Source: CAD feature listing. Evaluate the final solid. Frame: model axes, mm. A direction names the side the tool comes from. Give positions to 0.01 mm unless a question says otherwise; leave off trailing zeros. Write each loop counter-clockwise with the first axis right and the second up, starting at its lowest first coordinate (ties: lowest second). Pieces come first, ordered by that corner, then holes. Notation, with made-up numbers: (13.25, -25) - (60.25, -25) arc R25 ccw to (60.25, -3) - close; hole circle Ø7 at (46.25, -13). An arc over 180 degrees is marked (long way). One line per question, with ' | ' between items. Start each with the question number.
(1) Section A-A, the plane y = 6.25. Return loops of the section in (x, z), plus the area to 3 significant figures.
(2) Ray query, line 1 (Y direction, x = -7.75, z = 4); line 2 (Z direction, x = 0, y = 16.25); line 3 (Y direction, x = 1.75, z = 1.25). Return the intervals inside material, ascending. Write a range as [from, to].
(3) Access query for faces 1 (the cylindrical face through (-6, 16, 0)), 2 (the flat face through (0, 5.8, 7)), 3 (the cylindrical face through (-1.4, 22.34, -6.32)), 4 (the flat face through (6, 24.3, -2)). Directions: +Z, -Z, +X, -X, +Y, -Y. A direction counts if a zero-diameter tool reaches every point of the face in a straight line with its end or side. Return the directions, or none.
(4) Pin query (flat end, axial travel): pin 1 (5 mm diameter, centred on x = -7, y = 17, fed in from -Z); pin 2 (3.5 mm diameter, centred on x = -0.5, z = -2, fed in from +Y); pin 3 (2 mm diameter, centred on y = 8, z = 1.5, fed in from +X). Return the tip coordinate at first contact, or that it passes through.
(5) Draft query along X for faces 5 (the flat face through (-1.4, 7.3, 4.1)), 6 (the flat face through (0, -4.7, 0)), 7 (the conical face through (-5.24, 0.62, 4.01)). Return one class per face: +X half, -X half, draft (parallel to the pull), parting line (faces both ways), or undercut.
(6) Section C-C, the plane y = 13.25. Return loops of the section in (x, z), plus the area to 3 significant figures.
(7) Section B-B, the plane z = 0. Return loops of the section in (x, y) (3 decimals), plus the area to 3 significant figures.
Autodesk Inventor part; units mm, degrees
ref_plane "CNS_SCREW_XY" through (0, 0, 0) normal (0, 1, 0) x (1, 0, 0)
ref_plane "CNS_SCREW_YZ" through (0, 0, 0) normal (1, 0, 0) x (0, 0, -1)
ref_plane "CNS_SCREW_ZX" through (0, 0, 0) normal (0, 0, -1) x (0, 1, 0)
sketch "Sketch_1" plane through (0, 0, 0) normal (0, 0, 1) x (1, 0, 0)
  line L0 (0, -6.01) -> (0, 24.3)
  line L1 (0, 24.3) -> (9.1, 24.3)
  line L2 (9.1, 24.3) -> (9.1, 22.8)
  line L3 (9.1, 22.8) -> (6.475, 22.8)
  line L4 (6.475, 22.8) -> (6.475, 21.9)
  line L5 (6.475, 21.9) -> (9.1, 21.9)
  line L6 (9.1, 21.9) -> (9.1, 5.8)
  line L7 (9.1, 5.8) -> (6.7596, 5.8)
  line L8 (6.7596, 5.8) -> (6.3909, -6.01)
  line L9 (6.3909, -6.01) -> (0, -6.01)
  line L10 (0, -6.01) -> (0, 24.3)
revolve "Revolution1" add sketch "Sketch_1" angle 360 about axis through (0, -6.01, 0) along (0, -1, 0)
thread "Thread1"
sketch "_____1" plane through (0, 0, 0) normal (0, 0, 1) x (1, 0, 0)
  line L0 (-13.157, -4.7) -> (-13.157, -6.01)
  line L1 (-13.157, -6.01) -> (13.157, -6.01)
  line L2 (13.157, -6.01) -> (13.157, -4.7)
  line L3 (13.157, -4.7) -> (-13.157, -4.7)
extrude "Extrusion1" cut sketch "_____1" along normal mid plane 26.314
sketch "Sketch_2" plane through (0, 0, 0) normal (0, 0, 1) x (1, 0, 0)
  line L0 (0, 7.3) -> (0, 24.3)
  line L1 (0, 24.3) -> (6, 24.3)
  line L2 (6, 24.3) -> (6, 7.3)
  line L3 (6, 7.3) -> (0, 7.3)
  line L4 (0, 7.3) -> (0, 24.3)
revolve "Revolution2" cut sketch "Sketch_2" angle 360 about axis through (0, 7.3, 0) along (0, -1, 0)
sketch "Sketch_3" plane through (0, 24.3, 0) normal (0, 1, 0) x (1, 0, 0)
  line L0 (-4, -2.3094) -> (0, -4.6188)
  line L1 (0, -4.6188) -> (4, -2.3094)
  line L2 (4, -2.3094) -> (4, 2.3094)
  line L3 (4, 2.3094) -> (0, 4.6188)
  line L4 (0, 4.6188) -> (-4, 2.3094)
  line L5 (-4, 2.3094) -> (-4, -2.3094)
extrude "Extrusion2" cut sketch "Sketch_3" against normal blind 21.5
ref_plane "CNS_SCREW_XY" through (0, 0, 0) normal (0, 1, 0) x (1, 0, 0)
ref_plane "CNS_SCREW_YZ" through (0, 0, 0) normal (1, 0, 0) x (0, 0, -1)
ref_plane "CNS_SCREW_ZX" through (0, 0, 0) normal (0, 0, -1) x (0, 1, 0)
properties part number "KQ2S12-02AS (A) Brass"
Check sheet entries:
1) outline: circle Ø18.2 at (0, 0); hole (-4, -2.31) - (0, -4.62) - (4, -2.31) - (4, 2.31) - (0, 4.62) - (-4, 2.31) - close | area: 205 mm²
2) line 1: [5.8, 21.9], [22.8, 24.3] | line 2: [-9.1, -6], [6, 9.1] | line 3: [-4.7, 2.8]
3) face 1: +Y | face 2: -Y | face 3: none | face 4: +Z, -Z, +X, -X, +Y
4) pin 1: z = -7.91 | pin 2: y = 2.8 | pin 3: x = 9.09
5) face 5: undercut | face 6: draft | face 7: parting line
6) outline: circle Ø18.2 at (0, 0); hole circle Ø12 at (0, 0) | area: 147 mm²
7) outline: (-9.1, 5.8) - (-6.76, 5.8) - (-6.432, -4.7) - (6.432, -4.7) - (6.76, 5.8) - (9.1, 5.8) - (9.1, 21.9) - (6.475, 21.9) - (6.475, 22.8) - (9.1, 22.8) - (9.1, 24.3) - (6, 24.3) - (6, 7.3) - (4, 7.3) - (4, 2.8) - (-4, 2.8) - (-4, 7.3) - (-6, 7.3) - (-6, 24.3) - (-9.1, 24.3) - (-9.1, 22.8) - (-6.475, 22.8) - (-6.475, 21.9) - (-9.1, 21.9) - close | area: 230 mm²
